from build123d import *

# Parameters (mm, degrees)
SKETCH_1_R          = 12.2
EXTRUDE_1_DEPTH     = 35
SKETCH_2_R          = 6.5
EXTRUDE_2_DEPTH     = 2.6
EXTRUDE_3_DEPTH     = 14.4
CUT_EXTRUDE_START   = -1
SKETCH_4_R          = 6.5
SKETCH_4_R_2        = 6
CUT_EXTRUDE_2_DEPTH = 1
SKETCH_5_R          = 1.5
CUT_EXTRUDE_3_DEPTH = 56.397924149
SKETCH_6_R          = 1.5
CUT_EXTRUDE_5_DEPTH = 4


with BuildPart() as part:
    # 草图1 → 凸台-拉伸1 (new body)
    with BuildSketch(Plane.XY):
        Circle(SKETCH_1_R)
    extrude(amount=EXTRUDE_1_DEPTH)

    # 草图2 → 凸台-拉伸2 (add)
    with BuildSketch(Plane.XY.offset(35)):
        Circle(SKETCH_2_R)
    extrude(amount=EXTRUDE_2_DEPTH)

    # 草图3 → 凸台-拉伸3 (add)
    with BuildSketch(Plane.XY.offset(37.6)):
        with BuildLine():
            Line((-2.5, 1.658312395), (-2.5, -1.658312395))
            ThreePointArc((-2.5, -1.658312395), (3, 0), (-2.5, 1.658312395))
        make_face()
    extrude(amount=EXTRUDE_3_DEPTH)

    # 草图4 → 切除-拉伸2 (cut)
    with BuildSketch(Plane.XY.offset(37.6).offset(CUT_EXTRUDE_START)):
        Circle(SKETCH_4_R)
        Circle(SKETCH_4_R_2, mode=Mode.SUBTRACT)
    extrude(amount=CUT_EXTRUDE_2_DEPTH, mode=Mode.SUBTRACT)

    # 草图5 → 切除-拉伸3 (cut, through all)
    with BuildSketch(Plane.ZY.offset(2.5)):
        with Locations((43, 0)):
            Circle(SKETCH_5_R)
    extrude(amount=-CUT_EXTRUDE_3_DEPTH, mode=Mode.SUBTRACT)

    # 草图6 → 切除-拉伸5 (cut)
    with BuildSketch(Plane.XY.offset(35)):
        with Locations((0, 9.5)):
            Circle(SKETCH_6_R)
        with Locations((8.227241336, -4.75)):
            Circle(SKETCH_6_R)
        with Locations((-8.227241336, -4.75)):
            Circle(SKETCH_6_R)
    extrude(amount=-CUT_EXTRUDE_5_DEPTH, mode=Mode.SUBTRACT)


solid = part.part
Could you check a few things on this model? Use its own coordinates, in mm. A direction names the side the tool comes from. Coordinates: 2 decimals unless noted, no trailing zeros. Write each loop counter-clockwise with the first axis right and the second up, starting at its lowest first coordinate (ties: lowest second). Pieces come first, ordered by that corner, then holes. Notation, with made-up numbers: (73.25, 29) - (106.25, 29) arc R29 cw to (106.25, 56) - close; hole circle Ø5 at (72.25, 32). An arc over 180 degrees is marked (long way). Put each result on its own line as item: value. Start each with the question number.
Q1. I'm going to push flat-ended pins straight in: P1, Ø3.5, axis at x = 0, y = 9.5, coming from the +Z side; P2, Ø2.5, axis at x = -8.23, y = -4.75, coming from the +Z side; P3, Ø6, axis at x = -4, z = 27.5, coming from the -Y side; P4, Ø1.8, axis at y = 0, z = 43, coming from the +X side. Where does each tip first touch, or does it pass through?
Q2. I want a section at A-A on y = 0. Write out the boundary of the cut face in (x, z), plus the area to 4 significant figures.
Q3. I want a section at C-C on z = 43. Write out the boundary of the cut face in (x, y).
Q4. Please list where these lines run through material, in increasing order: L1, parallel to Z at x = -0.55, y = 0; L2, parallel to Z at x = 10.5, y = 5.75; L3, parallel to Z at x = -8, y = -4.25.
Q5. I want a section at B-B on x = 0. Write out the boundary of the cut face in (y, z), plus the area to 3 significant figures.
Q6. Which directions (+Z, -Z, +X, -X, +Y, -Y) give clear straight access to the entire face, cutting with the end or side of a thin tool? Please do faces 1 (the cylindrical face through (3, 0, 45)), 2 (the flat face through (0, 0, 52)).
Q7. Thinking about a two-plate mould opening in Y: for faces 3 (the cylindrical face through (0.21, 0.45, 44.43)), 4 (the cylindrical face through (9.66, -4.3, 33.03)), 5 (the flat face through (-2.5, 0, 45)), 6 (the cylindrical face through (-12.19, 0.54, 17.26)), which applies, pulls with the +Y half, pulls with the -Y half, needs draft (parallel to the pull), parting line crosses it, or undercut?
Q8. I want a section at D-D on z = 29. Write out the boundary of the cut face in (x, y).
Checks:
1. P1: z = 35
1. P2: z = 31
1. P3: y = -12.16
1. P4: through
2. outline: (-12.2, 0) - (12.2, 0) - (12.2, 35) - (6.5, 35) - (6.5, 36.6) - (6, 36.6) - (6, 37.6) - (3, 37.6) - (3, 41.5) - (-2.5, 41.5) - (-2.5, 37.6) - (-6, 37.6) - (-6, 36.6) - (-6.5, 36.6) - (-6.5, 35) - (-12.2, 35) - close; (-2.5, 44.5) - (3, 44.5) - (3, 52) - (-2.5, 52) - close
2. area: 949.5 mm²
3. outline: (-2.5, -1.66) arc R3 ccw to (2.6, -1.5) - (-2.5, -1.5) - close; (-2.5, 1.5) - (2.6, 1.5) arc R3 ccw to (-2.5, 1.66) - close
4. L1: 0 to 41.5, 44.5 to 52
4. L2: 0 to 35
4. L3: 0 to 31
5. outline: (-12.2, 0) - (12.2, 0) - (12.2, 35) - (11, 35) - (11, 31) - (8, 31) - (8, 35) - (6.5, 35) - (6.5, 36.6) - (6, 36.6) - (6, 37.6) - (3, 37.6) - (3, 52) - (-3, 52) - (-3, 37.6) - (-6, 37.6) - (-6, 36.6) - (-6.5, 36.6) - (-6.5, 35) - (-12.2, 35) - close; hole circle Ø3 at (0, 43)
5. area: 954 mm²
6. face 1: +Z
6. face 2: +Z, +X, -X, +Y, -Y
7. face 3: undercut
7. face 4: undercut
7. face 5: needs draft
7. face 6: parting line crosses it
8. outline: circle Ø24.4 at (0, 0)
